The listing builds one solid part. Answer for the finished solid, in the listing's coordinates (mm). Round coordinates to 2 decimals unless told otherwise and drop trailing zeros. Write each loop counter-clockwise with the first axis right and the second up, starting at its lowest first coordinate (ties: lowest second). Pieces come first, ordered by that corner, then holes. Notation, with made-up numbers: (39.25, 26.5) - (59.25, 26.5) arc R10 ccw to (59.25, 39.5) - close; hole circle Ø7 at (5, -36). An arc over 180 degrees is marked (long way). Return JSON: item names as keys, results as strings. Group by question number.
(1) Section A-A, the plane x = 19 is taken. Write down the section's boundary in (y, z).
(2) Determine the mould class of faces 1 (the flat face through (19, 0, 11)), 2 (the cylindrical face through (37.797, -0.246, 1.141)), 3 (the cylindrical face through (19.1, -0.2, 22)), 4 (the cylindrical face through (18.783, -0.246, 17.024)) for opening direction X: +X half, -X half, draft (parallel to the pull), parting line (faces both ways), or undercut.
(3) Each of these flat-tipped pins is pushed along its axis until it touches: pin 1 (8 mm diameter, centred on x = 21.5, z = 8.5, fed in from +Y); pin 2 (1.8 mm diameter, centred on x = 19, z = 18, fed in from +Y). Where does it stop, or does it pass through?
(4) Section C-C, the plane z = 18.5 is taken. Write down the section's boundary in (x, y).
(5) Find the intervals of material crossed by line 1 along Z through (x, y) = (19, -0.15); line 2 along Z through (x, y) = (31.5, -0.25); line 3 along Z through (x, y) = (22, -0.2), in increasing order. Write a range as [from, to].
(6) Section D-D, the plane x = 31.5 is taken. Write down the section's boundary in (y, z).
(7) Section B-B, the plane y = -0.25 is taken. Write down the section's boundary in (x, z), then the cut area to 3 significant figures.
```python
from build123d import *

# Parameters (mm, degrees)
F0_R     = 1
F1_DEPTH = 0.5


with BuildPart() as f1:
    # F0 (on Front) → F1 (new body)
    with BuildSketch(Plane.XZ):
        with BuildLine():
            ThreePointArc((0, 4), (1.171573, 1.171573), (4, 0))
            Line((4, 0), (35, 0))
            ThreePointArc((35, 0), (37.828427, 1.171573), (39, 4))
            Line((39, 4), (39, 17.908077))
            ThreePointArc((39, 17.908077), (37.508278, 18.476782), (36, 19))
            Line((36, 19), (27.660254, 19))
            ThreePointArc((27.660254, 19), (26.02362, 19.275444), (24.567306, 20.071429))
            ThreePointArc((24.567306, 20.071429), (19, 22), (13.432694, 20.071429))
            ThreePointArc((13.432694, 20.071429), (11.97638, 19.275444), (10.339746, 19))
            Line((10.339746, 19), (3, 19))
            ThreePointArc((3, 19), (1.491722, 18.476782), (0, 17.908077))
            Line((0, 17.908077), (0, 4))
        make_face()
        with Locations((19, 18)):
            Circle(F0_R, mode=Mode.SUBTRACT)
    extrude(amount=F1_DEPTH)


solid = f1.part
```
Working result:
{
 "1": {"outline": "(-0.5, 0) - (0, 0) - (0, 17) - (-0.5, 17) - close; (-0.5, 19) - (0, 19) - (0, 22) - (-0.5, 22) - close"},
 "2": {"face 1": "draft", "face 2": "+X half", "face 3": "parting line", "face 4": "undercut"},
 "3": {"pin 1": "stops at y = 0", "pin 2": "passes through"},
 "4": {"outline": "(1.56, -0.5) - (18.13, -0.5) - (18.13, 0) - (1.56, 0) - close; (19.87, -0.5) - (37.44, -0.5) - (37.44, 0) - (19.87, 0) - close"},
 "5": {"line 1": "z = [0, 17], [19, 22]", "line 2": "z = [0, 19]", "line 3": "z = [0, 21.49]"},
 "6": {"outline": "(-0.5, 0) - (0, 0) - (0, 19) - (-0.5, 19) - close"},
 "7": {"outline": "(0, 4) arc R4 ccw to (4, 0) - (35, 0) arc R4 ccw to (39, 4) - (39, 17.91) arc R52.65 ccw to (36, 19) - (27.66, 19) arc R5 cw to (24.57, 20.07) arc R9 ccw to (13.43, 20.07) arc R5 cw to (10.34, 19) - (3, 19) arc R52.65 ccw to (0, 17.91) - close; hole circle Ø2 at (19, 18)", "area": "757 mm^2"}
}
